Autodesk Inventor part; units mm, degrees
ref_plane "YZ Plane" through (0, 0, 0) normal (1, 0, 0) x (0, 1, 0)
ref_plane "XZ Plane" through (0, 0, 0) normal (0, 1, 0) x (-1, 0, 0)
ref_plane "XY Plane" through (0, 0, 0) normal (0, 0, 1) x (1, 0, 0)
sketch "Sketch1" plane through (0, 0, 0) normal (0, 0, 1) x (1, 0, 0)
  line L0 (0, 0) -> (250, 0)
  line L1 (250, 0) -> (250, 150)
  line L2 (0, 150) -> (0, 0)
  line L3 (0, 150) -> (80, 350)
  line L4 (80, 350) -> (80, 600)
  line L5 (280, 600) -> (280, 230)
  line L6 (250, 150) -> (250, 200)
  line L7 (250, 200) -> (280, 230)
  line L8 (80, 600) -> (280, 600)
  dimension "d0" = 250
  dimension "d1" = 150
  dimension "d3" = 80
  dimension "d5" = 30
  dimension "d6" = 50
  dimension "d8" = 600
  dimension "d9" = 200
  dimension "d10" = 30
  dimension "d11" = 150
extrude "Extrusion1" add sketch "Sketch1" along normal blind 16
fillet "Fillet1" radius 10 4 edges at (80, 600, 8) (280, 600, 8) (0, 0, 8) (250, 0, 8)
sketch "Sketch9" plane through (0, 0, 16) normal (0, 0, 1) x (1, 0, 0)
  line L0 (0, 150) -> (0, 10)
  line L1 (0, 35) -> (250, 35)
  line L2 (250, 10) -> (250, 200)
  line L3 (10, 0) -> (240, 0)
  circle A0 centre (30, 35) radius 5
  circle A1 centre (69, 35) radius 5
  circle A2 centre (181, 35) radius 5
  circle A3 centre (220, 35) radius 5
  line L4 (25, 35) -> (25, 55)
  line L5 (35, 35) -> (35, 55)
  circle A4 centre (30, 55) radius 5
  circle A5 centre (69, 55) radius 5
  line L6 (64, 55) -> (64, 35)
  line L7 (74, 55) -> (74, 35)
  line L8 (0, 100) -> (250, 100)
  circle A6 centre (125, 50) radius 5
  circle A7 centre (220, 55) radius 5
  line L9 (215, 55) -> (215, 35)
  line L10 (225, 55) -> (225, 35)
  circle A8 centre (181, 55) radius 5
  line L11 (176, 55) -> (176, 35)
  line L12 (186, 55) -> (186, 35)
  point P0 (0, 0)
  point P1 (0, 148.0742)
  point P2 (250, 196.6667)
  point P3 (125, 100)
  dimension "d111" = 35
  dimension "d112" = 30
  dimension "d113" = 10
  dimension "d114" = 20
  dimension "d116" = 10
  dimension "d117" = 10
  dimension "d118" = 10
  dimension "d119" = 20
  dimension "d120" = 100
  dimension "d121" = 10
  dimension "d122" = 50
  dimension "d123" = 30
  dimension "d124" = 20
  dimension "d127" = 29
  dimension "d128" = 29
  dimension "d129" = 20
  dimension "d153" = 10
  dimension "d154" = 0
  dimension "d155" = 10
  dimension "d156" = 10
  dimension "d157" = 10
extrude "Extrusion7" cut sketch "Sketch9" against normal through all contours A0 L1 | L4 A4 L5 A0 | L1 A0 | A4 | A3 L1 | L1 A3 | A3 L9 A7 L10 | A1 L1 | L6 A5 L7 A1 | L1 A1 | A7 | A5 | A2 L1 | L1 A2 | A2 L11 A8 L12 | A8
sketch "Sketch10" plane through (0, 0, 0) normal (0, 0, -1) x (-1, 0, 0)
  line L0 (-280, 230) -> (-280, 590)
  line L1 (-280, 560) -> (-80, 560)
  line L2 (-80, 590) -> (-80, 350)
  line L3 (-270, 600) -> (-90, 600)
  line L4 (-270, 600) -> (-90, 600)
  line L5 (-180, 600) -> (-180, 520)
  line L6 (-200, 580) -> (-160, 580)
  line L7 (-160, 580) -> (-160, 540)
  line L8 (-160, 540) -> (-200, 540)
  line L9 (-200, 540) -> (-200, 580)
  line L10 (-200, 580) -> (-160, 540) construction
  line L11 (-160, 580) -> (-200, 540) construction
  circle A0 centre (-200, 560) radius 4.5
  circle A1 centre (-160, 560) radius 4.5
  circle A2 centre (-260, 560) radius 4.5
  circle A3 centre (-100, 560) radius 4.5
  line L12 (-180, 520) -> (-180, 380)
  line L13 (-200, 400) -> (-160, 400)
  line L14 (-160, 400) -> (-160, 360)
  line L15 (-160, 360) -> (-200, 360)
  line L16 (-200, 360) -> (-200, 400)
  line L17 (-200, 400) -> (-160, 360) construction
  line L18 (-160, 400) -> (-200, 360) construction
  line L19 (-280, 380) -> (-80, 380)
  circle A4 centre (-260, 380) radius 4.5
  circle A5 centre (-100, 380) radius 4.5
  circle A6 centre (-200, 380) radius 4.5
  circle A7 centre (-160, 380) radius 4.5
  point P0 (0, 0)
  point P1 (-280, 243.3333)
  point P2 (-80, 351.9258)
  point P3 (-180, 560)
  dimension "d130" = 40
  dimension "d131" = 80
  dimension "d132" = 40
  dimension "d133" = 40
  dimension "d134" = 9
  dimension "d135" = 9
  dimension "d136" = 9
  dimension "d137" = 9
  dimension "d138" = 60
  dimension "d139" = 60
  dimension "d140" = 140
  dimension "d141" = 40
  dimension "d142" = 40
  dimension "d143" = 9
  dimension "d144" = 220
  dimension "d145" = 9
  dimension "d146" = 9
  dimension "d147" = 9
  dimension "d148" = 60
  dimension "d149" = 60
extrude "Extrusion8" cut sketch "Sketch10" against normal through all contours A4 L19 | L19 A4 | A2 L1 | L1 A2 | A6 L16 L19 | L19 L16 A6 | A0 L9 L1 | L1 L9 A0 | L19 A6 L16 | L16 A6 L19 | L9 A0 L1 | L1 A0 L9 | A7 L14 L19 | L19 L14 A7 | L14 L19 A7 | A1 L7 L1 | L1 L7 A1 | L14 A7 L19 | L7 A1 L1 | L1 A1 L7 | A5 L19 | L19 A5 | A3 L1 | L1 A3
fillet "Fillet3" radius 5 4 edges at (280, 230, 8) (250, 200, 8) (0, 150, 8) (80, 350, 8)
properties part number "PA1"
The model under review builds one solid part; all positions refer to its coordinate system, in mm. A direction names the side the tool comes from. Coordinates: 2 decimals unless noted, no trailing zeros. Write each loop counter-clockwise with the first axis right and the second up, starting at its lowest first coordinate (ties: lowest second). Pieces come first, ordered by that corner, then holes.
1) The part is to be moulded in two halves that separate along X. For faces 1 (the face through (265, 215, 8)), 2 (the face through (179, 600, 8)), 3 (the face through (0, 80, 8)), 4 (the face through (74, 45, 8)), say which applies: pulls with the +X half, pulls with the -X half, needs draft (parallel to the pull), parting line crosses it, or undercut.
2) Machinability: for faces 5 (the face through (2.85, 3.01, 8.11)), 6 (the face through (80, 469, 8)), 7 (the face through (123, 0, 8)), 8 (the face through (250, 103, 8)), 9 (the face through (186, 45, 8)), which of the approach directions +Z, -Z, +X, -X, +Y, -Y give a long, thin tool a straight path to every point of the face, cutting with its end or side? Answer none if there is none.
3) Clearance check with flat-ended pins moving along their axes: pin 1 Ø10.5 at (x, y) = (100, 560) entering from -Z; pin 2 Ø4 at (y, z) = (286.5, 8) entering from -X; pin 3 Ø3 at (y, z) = (507, 9.5) entering from -X; pin 4 Ø5 at (y, z) = (49, 8) entering from +X. State where each tip first meets the part, or that it passes through.
4) To check wall thickness, follow probe 1 along X at (y, z) = (560, 12); probe 2 along Y at (x, z) = (99, 7.75); probe 3 along Y at (x, z) = (257.5, 11.75). State the ranges of each line that lie inside material, in increasing order.
5) We need section A-A on z = 10.75. Count the separate pieces of the cut face and the enclosed holes in it, then the cut area to 3 significant figures.
6) We need section B-B on x = 57. State the section outline as (y, z) points, then the cut area to 3 significant figures.
7) We need section C-C on y = 314.5. State the section outline as (x, z) points, then the cut area to 3 significant figures.
Answer list:
1. face 1: pulls with the +X half
1. face 2: needs draft
1. face 3: pulls with the -X half
1. face 4: undercut
2. face 5: +Z, -Z, -X, -Y
2. face 6: +Z, -Z, -X, +Y
2. face 7: +Z, -Z, +X, -X, -Y
2. face 8: +Z, -Z, +X, -Y
2. face 9: +Z, -Z
3. pin 1: stops at z = 0
3. pin 2: stops at x = 53.8
3. pin 3: stops at x = 80
3. pin 4: stops at x = 250
4. probe 1: x = 80 to 95.5, 104.5 to 155.5, 164.5 to 195.5, 204.5 to 255.5, 264.5 to 280
4. probe 2: y = 0 to 375.61, 384.39 to 555.61, 564.39 to 600
4. probe 3: y = 207.5 to 376.26, 383.74 to 556.26, 563.74 to 600
5. separate pieces: 1
5. enclosed holes: 12
5. area: 132,000 mm2
6. outline: (0, 0) - (292.5, 0) - (292.5, 16) - (0, 16) - close
6. area: 4,680 mm2
7. outline: (65.8, 0) - (280, 0) - (280, 16) - (65.8, 16) - close
7. area: 3,430 mm2
